```python
from build123d import *

# Parameters (mm, degrees)
EXTRUDE_1_DEPTH     = 15
SKETCH_2_R          = 33
EXTRUDE_2_DEPTH     = 50
SKETCH_3_RX         = 60
SKETCH_3_RY         = 37.5
EXTRUDE_3_DEPTH     = 15
SKETCH_4_R          = 21
CUT_EXTRUDE_1_DEPTH = 65
CUT_EXTRUDE_2_REACH = 119.606
SKETCH_5_R          = 16.5
CUT_EXTRUDE_3_REACH = 119.606
SKETCH_6_R          = 5.4
FILLET_1_R          = 5


with BuildPart() as part:
    # 草图1 → 凸台-拉伸1 (new body)
    with BuildSketch(Plane(origin=(0, 0, 0), x_dir=(1, 0, 0), z_dir=(0, 1, 0))):
        with BuildLine():
            Line((-70, -42.5), (70, -42.5))
            ThreePointArc((70, -42.5), (73.535533906, -41.035533906), (75, -37.5))
            Line((75, -37.5), (75, 37.5))
            ThreePointArc((75, 37.5), (73.535533906, 41.035533906), (70, 42.5))
            Line((70, 42.5), (-70, 42.5))
            ThreePointArc((-70, 42.5), (-73.535533906, 41.035533906), (-75, 37.5))
            Line((-75, 37.5), (-75, -37.5))
            ThreePointArc((-75, -37.5), (-73.535533906, -41.035533906), (-70, -42.5))
        make_face()
    extrude(amount=EXTRUDE_1_DEPTH)

    # 草图2 → 凸台-拉伸2 (add)
    with BuildSketch(Plane(origin=(0, 15, 0), x_dir=(1, 0, 0), z_dir=(0, 1, 0))):
        with Locations(Location((0, 0, 0), (0, 0, 90))):
            Circle(SKETCH_2_R)
    extrude(amount=EXTRUDE_2_DEPTH)

    # 草图3 → 凸台-拉伸3 (add)
    with BuildSketch(Plane(origin=(0, 65, 0), x_dir=(1, 0, 0), z_dir=(0, 1, 0))):
        with Locations((0, 0)):
            Ellipse(SKETCH_3_RX, SKETCH_3_RY)
    extrude(amount=EXTRUDE_3_DEPTH)

    # 草图4 → 切除-拉伸1 (cut)
    with BuildSketch(Plane(origin=(0, 80, 0), x_dir=(1, 0, 0), z_dir=(0, 1, 0))):
        with Locations(Location((0, 0, 0), (0, 0, 270))):
            Circle(SKETCH_4_R)
    extrude(amount=-CUT_EXTRUDE_1_DEPTH, mode=Mode.SUBTRACT)

    # 草图5 → 切除-拉伸2 (cut, up to next)
    with BuildSketch(Plane.XZ, mode=Mode.PRIVATE) as cut_extrude_2_sk1:
        with Locations(Location((0, 0, 0), (0, 0, 270))):
            Circle(SKETCH_5_R)
    cut_extrude_2_tool1 = extrude(cut_extrude_2_sk1.sketch, amount=-CUT_EXTRUDE_2_REACH, mode=Mode.PRIVATE) & part.part
    add(cut_extrude_2_tool1.solids().sort_by_distance((0, 0, 0))[0], mode=Mode.SUBTRACT)

    # 草图6 → 切除-拉伸3 (cut, up to next)
    with BuildSketch(Plane(origin=(0, 80, 0), x_dir=(1, 0, 0), z_dir=(0, 1, 0)), mode=Mode.PRIVATE) as cut_extrude_3_sk1:
        with Locations(Location((42, 0, 0), (0, 0, 270))):
            Circle(SKETCH_6_R)
    cut_extrude_3_tool1 = extrude(cut_extrude_3_sk1.sketch, amount=-CUT_EXTRUDE_3_REACH, mode=Mode.PRIVATE) & part.part
    # 草图6 → 切除-拉伸3 (cut, up to next)
    with BuildSketch(Plane(origin=(0, 80, 0), x_dir=(1, 0, 0), z_dir=(0, 1, 0)), mode=Mode.PRIVATE) as cut_extrude_3_sk2:
        with Locations(Location((-42, 0, 0), (0, 0, 270))):
            Circle(SKETCH_6_R)
    cut_extrude_3_tool2 = extrude(cut_extrude_3_sk2.sketch, amount=-CUT_EXTRUDE_3_REACH, mode=Mode.PRIVATE) & part.part
    add(cut_extrude_3_tool1.solids().sort_by_distance((42, 80, 0))[0], mode=Mode.SUBTRACT)
    add(cut_extrude_3_tool2.solids().sort_by_distance((-42, 80, 0))[0], mode=Mode.SUBTRACT)

    # 圆角1
    fillet_1_edges = [part.edges().sort_by_distance(p)[0] for p in [
        (0, 15, 33),
    ]]
    fillet(fillet_1_edges, radius=FILLET_1_R)


solid = part.part
```
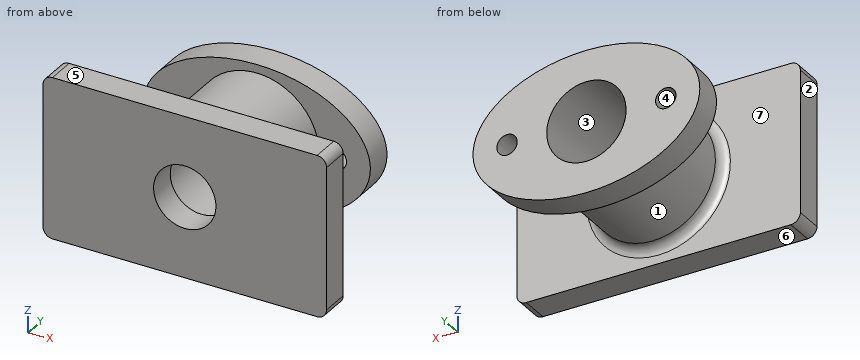
Verification items for the finished model (mm, model axes). Face numbers are marked on the shaded views. A direction names the side the tool comes from. Coordinates: 2 decimals unless noted, no trailing zeros. Write each loop counter-clockwise with the first axis right and the second up, starting at its lowest first coordinate (ties: lowest second). Pieces come first, ordered by that corner, then holes. Notation, with made-up numbers: M 50,61.25 L 77,61.25 A30 cw 77,94.25 Z; hole C -25,76 d1. An arc over 180 degrees is marked long. One line per item, written item: value.
Item 1: Gauge pin test, flat ends, axial feed: pin 1 Ø10 at (y, z) = (19, -21) entering from -X; pin 2 Ø8 at (y, z) = (60, -8.5) entering from -X; pin 3 Ø1 at (y, z) = (24, 12) entering from +X; pin 4 Ø9.5 at (x, z) = (42, 0) entering from +Y. Record the tip position at first contact, or that the pin passes through.
Check sheet entries:
pin 1: stops at x = -75
pin 2: stops at x = -32.69
pin 3: stops at x = 30.93
pin 4: stops at y = 15.06
Item 2: Scan lines: line 1 along X through (y, z) = (76, 0); line 2 along Y through (x, z) = (-54.5, 5.5); line 3 along X through (y, z) = (76.5, -3). Record each from-to range of solid material in increasing order.
Check sheet entries:
line 1: x = -60 to -47.4, -36.6 to -21, 21 to 36.6, 47.4 to 60
line 2: y = 0 to 15, 65 to 80
line 3: x = -59.81 to -46.49, -37.51 to -20.78, 20.78 to 37.51, 46.49 to 59.81
Item 3: Mould release check, pull along Z, two halves, no side actions. Record for the marked faces 4, 5, 6 and 7: pulls with the +Z half, pulls with the -Z half, needs draft (parallel to the pull), parting line crosses it, or undercut.
Check sheet entries:
face 4: undercut
face 5: pulls with the +Z half
face 6: pulls with the -Z half
face 7: needs draft
Item 4: Section check D-D, the plane y = 29. Record the boundary of the cut face in (x, z), plus the area to 3 significant figures.
Check sheet entries:
outline: C 0,0 d66; hole C 0,0 d42
area: 2,040 mm^2
Item 5: Access from +Z, -Z, +X, -X, +Y, -Y to the whole of each face (thin tool, end or side, straight path). Record for the marked faces 1, 2 and 3.
Check sheet entries:
face 1: none
face 2: +Z, -Z, -X, +Y, -Y
face 3: +Y
Item 6: Section check B-B, the plane z = 0. State how many separate pieces and enclosed holes the cut face has, plus the area to 3 significant figures.
Check sheet entries:
separate pieces: 4
enclosed holes: 0
area: 3,810 mm^2
Item 7: Section check C-C, the plane x = -63. Record the boundary of the cut face in (y, z), plus the area to 4 significant figures.
Check sheet entries:
outline: M 0,-42.5 L 15,-42.5 L 15,42.5 L 0,42.5 Z
area: 1,275 mm^2
Item 8: Section check A-A, the plane y = 9. Record the boundary of the cut face in (x, z), plus the area to 3 significant figures.
Check sheet entries:
outline: M -75,-37.5 A5 ccw -70,-42.5 L 70,-42.5 A5 ccw 75,-37.5 L 75,37.5 A5 ccw 70,42.5 L -70,42.5 A5 ccw -75,37.5 Z; hole C 0,0 d33
area: 11,900 mm^2
